Can you work these out from the model? Positions are in its coordinate system, mm. A direction names the side the tool comes from. Give positions to 0.01 mm unless a question says otherwise; leave off trailing zeros. Order: outer loops, then holes, each group sorted by start corner. A loop starts at its lowest first (then second) coordinate and runs counter-clockwise, first axis right, second up. Notation, with made-up numbers: (61.5, -10.5) -> (83.5, -10.5) arc R24 cw to (83.5, 2.5) -> close; hole circle Ø2 at (60.25, 5). An arc over 180 degrees is marked (long way). Answer as CSV lines item,"result".
```python
from build123d import *

# Parameters (mm, degrees)
F0_W     = 755
F0_H     = 755
F0_W_2   = 300
F0_H_2   = 300
F1_DEPTH = 30
F0_W_3   = 815
F0_H_3   = 815
F2_DEPTH = 60
F4_W     = 300
F4_H     = 300
F5_R     = 15.0176261861


with BuildPart() as f1:
    # F0 (on Top) → F1 (new body)
    with BuildSketch(Plane.XY):
        Rectangle(F0_W, F0_H)
        Rectangle(F0_W_2, F0_H_2, mode=Mode.SUBTRACT)
        Rectangle(F0_W_2, F0_H_2)
    extrude(amount=F1_DEPTH)

    # F0 (on Top) → F2 (join)
    with BuildSketch(Plane.XY):
        Rectangle(F0_W_3, F0_H_3)
        Rectangle(F0_W, F0_H, mode=Mode.SUBTRACT)
    extrude(amount=F2_DEPTH)

    # F4 (on face) → F6 section 0
    with BuildSketch(Plane.XY.offset(30)):
        Rectangle(F4_W, F4_H)
    # F5 (on offset) → F6 section 1
    with BuildSketch(Plane.XY.offset(430)):
        Circle(F5_R)
    loft()


solid = f1.part
```
Item 1: We'd pull the mould along X, two halves only. Please class faces 3 (the flat face through (-377.5, -5, 45)), 4 (the flat face through (-6, 407.5, 30)), 5 (the flat face through (-173, 5, 30)), 6 (the flat face through (-407.5, -6, 30)): released by +X, released by -X, zero draft, split by the parting line, or undercut.
Numbers:
face 3,"undercut"
face 4,"zero draft"
face 5,"undercut"
face 6,"released by -X"
Item 2: Please list where these lines run through material, in increasing order: line 1 along Y through (x, z) = (-349.5, 40); line 2 along Z through (x, y) = (126, 369); line 3 along Y through (x, z) = (143, 32).
Numbers:
line 1,"y = -407.5 to -377.5, 377.5 to 407.5"
line 2,"z = 0 to 30"
line 3,"y = -407.5 to -377.5, -149.3 to 149.3, 377.5 to 407.5"
Item 3: For pin 1 (5 mm diameter, centred on y = -0.5, z = 263.5, fed in from +X); pin 2 (6 mm diameter, centred on y = -81, z = 85, fed in from +X); pin 3 (4 mm diameter, centred on x = 229, y = -150, fed in from +Z), each with a flat end and sliding along its axis, tell me the tip position at first contact or that it passes through.
Numbers:
pin 1,"stops at x = 72.05"
pin 2,"stops at x = 132.23"
pin 3,"stops at z = 30"
Item 4: For faces 1 (the flat face through (-5, -377.5, 45)), 2 (the flat face through (-6, 6, 0)), which set-ups out of +Z, -Z, +X, -X, +Y, -Y let a thin tool reach every point of the face, with its end or its side?
Numbers:
face 1,"+Z"
face 2,"-Z, +X, -X, +Y, -Y"
Item 5: Imagine slicing it at A-A, the plane x = -187. Please give me the cut outline in (y, z), then the cut area to 4 significant figures.
Numbers:
outline,"(-407.5, 0) -> (407.5, 0) -> (407.5, 60) -> (377.5, 60) -> (377.5, 30) -> (-377.5, 30) -> (-377.5, 60) -> (-407.5, 60) -> close"
area,"26,250 mm²"
